```python
from build123d import *

# Parameters (mm, degrees)
SALIENTE_EXTRUIR1_DEPTH = 10
CROQUIS2_R              = 2.25
CORTAR_EXTRUIR1_DEPTH   = 11
CROQUIS3_R              = 2.25
CORTAR_EXTRUIR2_DEPTH   = 10
CROQUIS4_OUTSIDE_W      = 393.144
CROQUIS4_OUTSIDE_H      = 382.951
CROQUIS4_OUTSIDE_W_2    = 300
CROQUIS4_OUTSIDE_H_2    = 346.918637929
CORTAR_EXTRUIR3_DEPTH   = 10


with BuildPart() as part:
    # Croquis1 → Saliente-Extruir1 (new body)
    with BuildSketch(Plane.XY):
        with BuildLine():
            Line((303.558552598, 129.486748241), (275.155897415, 170.049943626))
            ThreePointArc((275.155897415, 170.049943626), (270.330951096, 174.281307983), (264.097344818, 175.806661735))
            Line((264.097344818, 175.806661735), (41.902655182, 175.806661735))
            ThreePointArc((41.902655182, 175.806661735), (35.669048904, 174.281307983), (30.844102585, 170.049943626))
            Line((30.844102585, 170.049943626), (2.441447402, 129.486748241))
            ThreePointArc((2.441447402, 129.486748241), (0.624821165, 125.802994643), (0, 121.74346635))
            Line((0, 121.74346635), (0, 0))
            Line((0, 0), (0, -120))
            Line((0, -120), (306, -120))
            Line((306, -120), (306, 0))
            Line((306, 0), (306, 121.74346635))
            ThreePointArc((306, 121.74346635), (305.375178835, 125.802994643), (303.558552598, 129.486748241))
        make_face()
        Polygon((20, 0), (20, 119.694024222), (45.286341011, 155.806661735), (260.713658989, 155.806661735), (286, 119.694024222), (286, 0), (286, -100), (20, -100), align=None, mode=Mode.SUBTRACT)
    extrude(amount=SALIENTE_EXTRUIR1_DEPTH)

    # Croquis2 → Cortar-Extruir1 (cut, through all)
    with BuildSketch(Plane.XY.offset(10)):
        with Locations((108, 163.806661735)):
            Circle(CROQUIS2_R)
        with Locations((198, 163.806661735)):
            Circle(CROQUIS2_R)
        with Locations((12, 10)):
            Circle(CROQUIS2_R)
        with Locations((294, 10)):
            Circle(CROQUIS2_R)
        with Locations((294, 90)):
            Circle(CROQUIS2_R)
        with Locations((12, 90)):
            Circle(CROQUIS2_R)
    extrude(amount=-CORTAR_EXTRUIR1_DEPTH, mode=Mode.SUBTRACT)

    # Croquis3 → Cortar-Extruir2 (cut)
    with BuildSketch(Plane.XY.offset(10)):
        with Locations((10, -35)):
            Circle(CROQUIS3_R)
        with Locations((296, -35)):
            Circle(CROQUIS3_R)
        with Locations((53, -110)):
            Circle(CROQUIS3_R)
        with Locations((153, -110)):
            Circle(CROQUIS3_R)
        with Locations((253, -110)):
            Circle(CROQUIS3_R)
    extrude(amount=-CORTAR_EXTRUIR2_DEPTH, mode=Mode.SUBTRACT)

    # Croquis4 outside → Cortar-Extruir3 (cut)
    with BuildSketch(Plane.XY.offset(10)):
        with Locations((153, 27.9035)):
            Rectangle(CROQUIS4_OUTSIDE_W, CROQUIS4_OUTSIDE_H)
        with Locations((153, 32.896001841)):
            Rectangle(CROQUIS4_OUTSIDE_W_2, CROQUIS4_OUTSIDE_H_2, mode=Mode.SUBTRACT)
    extrude(amount=-CORTAR_EXTRUIR3_DEPTH, mode=Mode.SUBTRACT)


solid = part.part
```
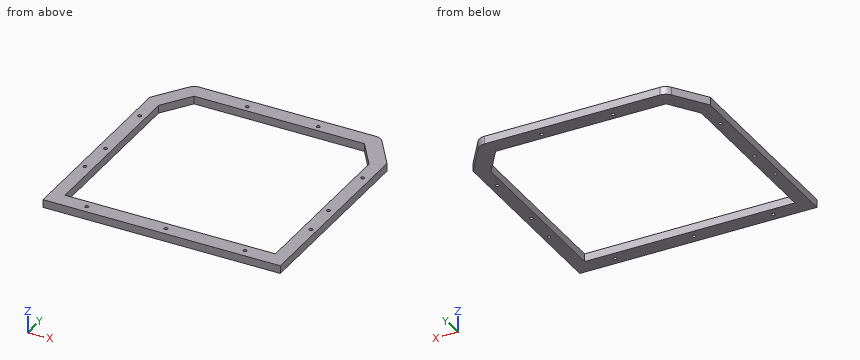
Can you work these out from the model? Positions are in its coordinate system, mm. Give positions to 0.01 mm unless a question says otherwise; leave off trailing zeros. Loops run counter-clockwise (first coordinate to the right, second up) from the corner with the lowest first, then second, coordinate; pieces in that order, holes last. Notation, with made-up numbers: M 79,67 L 87,67 A33 ccw 87,105 Z; hole C 44.25,-5.5 d2. An arc over 180 degrees is marked long. One line per item, written item: value.
(1) Suppose I cut it at B-B on x = 70.5. List the corners of the cut face in (y, z) for me.
Returned:
outline: M -120,0 L -100,0 L -100,10 L -120,10 Z; M 155.81,0 L 175.81,0 L 175.81,10 L 155.81,10 Z
(2) Will this pin go through, and if not, where does the flat tip stop? pin 1 (3.5 mm diameter, centred on x = 12, y = 10, fed in from +Z).
Returned:
pin 1: through
(3) Suppose I cut it at C-C on z = 5.5. Count the separate pieces of the cut face and the enclosed holes in it, plus the area to 3 significant figures.
Returned:
separate pieces: 1
enclosed holes: 12
area: 20,000 mm^2
(4) Suppose I cut it at A-A on y = -79. List the corners of the cut face in (x, z) for me, plus the area to 3 significant figures.
Returned:
outline: M 3,0 L 20,0 L 20,10 L 3,10 Z; M 286,0 L 303,0 L 303,10 L 286,10 Z
area: 340 mm^2
(5) I need wall thicknesses on line 1 (Y direction, x = 253, z = 4.5); line 2 (X direction, y = -47, z = 8); line 3 (Y direction, x = 139, z = 5.75). Which ranges of each line are inside material? Lowest first, please.
Returned:
line 1: -120 to -112.25, -107.75 to -100, 155.81 to 175.81
line 2: 3 to 20, 286 to 303
line 3: -120 to -100, 155.81 to 175.81
